from build123d import *

# Parameters (mm, degrees)
F0_W     = 15.85
F0_H     = 47.8
F1_DEPTH = 5
F2_R     = 2.5
F3_DEPTH = 2
F4_W     = 13.33
F4_H     = 44.9
F5_DEPTH = 2.8
F7_DEPTH = 2.8


with BuildPart() as f1:
    # F0 (on Top) → F1 (new body)
    with BuildSketch(Plane.XY):
        with Locations((-44.90279, 38.503254)):
            Rectangle(F0_W, F0_H)
    extrude(amount=F1_DEPTH)

    # F2 (on face) → F3 (join)
    with BuildSketch(Plane.XY.offset(5)):
        with Locations((-48.82779, 58.403254)):
            Circle(F2_R)
        with Locations((-40.97779, 58.403254)):
            Circle(F2_R)
        with Locations((-48.82779, 18.603254)):
            Circle(F2_R)
        with Locations((-40.97779, 18.603254)):
            Circle(F2_R)
        with Locations((-48.82779, 50.403254)):
            Circle(F2_R)
        with Locations((-40.97779, 50.403254)):
            Circle(F2_R)
        with Locations((-48.82779, 26.403254)):
            Circle(F2_R)
        with Locations((-40.97779, 26.403254)):
            Circle(F2_R)
        with Locations((-48.82779, 42.403254)):
            Circle(F2_R)
        with Locations((-40.97779, 42.403254)):
            Circle(F2_R)
        with Locations((-48.82779, 34.403254)):
            Circle(F2_R)
        with Locations((-40.97779, 34.403254)):
            Circle(F2_R)
    extrude(amount=F3_DEPTH)

    # F4 (on face) → F5 (cut)
    with BuildSketch(Plane(origin=(0, 0, 0), x_dir=(1, 0, 0), z_dir=(0, 0, -1))):
        with Locations((-44.856941, -38.523254)):
            Rectangle(F4_W, F4_H)
    extrude(amount=-F5_DEPTH, mode=Mode.SUBTRACT)

    # F6 (on face) → F7 (join)
    with BuildSketch(Plane(origin=(0, 0, 2.8), x_dir=(1, 0, 0), z_dir=(0, 0, -1))):
        with BuildLine():
            ThreePointArc((-41.606941, -21.923254), (-42.558844, -19.625157), (-44.856941, -18.673254))
            Line((-44.856941, -18.673254), (-44.856941, -19.873254))
            ThreePointArc((-44.856941, -19.873254), (-43.407372, -20.473685), (-42.806941, -21.923254))
            ThreePointArc((-42.806941, -21.923254), (-43.407372, -23.372823), (-44.856941, -23.973254))
            Line((-44.856941, -23.973254), (-44.856941, -25.173254))
            ThreePointArc((-44.856941, -25.173254), (-42.558844, -24.221351), (-41.606941, -21.923254))
        make_face()
        with BuildLine():
            ThreePointArc((-41.783448, -56.322801), (-42.673771, -54.08798), (-44.856941, -53.077598))
            Line((-44.856941, -53.077598), (-44.856941, -54.279652))
            ThreePointArc((-44.856941, -54.279652), (-43.516394, -54.933528), (-42.973804, -56.32285))
            ThreePointArc((-42.973804, -56.32285), (-43.516394, -57.712172), (-44.856941, -58.366047))
            Line((-44.856941, -58.366047), (-44.856941, -59.568005))
            ThreePointArc((-44.856941, -59.568005), (-42.673771, -58.557623), (-41.783448, -56.322801))
        make_face()
        with BuildLine():
            Line((-44.856941, -54.279652), (-44.856941, -53.077598))
            ThreePointArc((-44.856941, -53.077598), (-48.283448, -56.322801), (-44.856941, -59.568005))
            Line((-44.856941, -59.568005), (-44.856941, -58.366047))
            ThreePointArc((-44.856941, -58.366047), (-47.073804, -56.32285), (-44.856941, -54.279652))
        make_face()
        with BuildLine():
            ThreePointArc((-41.739321, -47.722915), (-42.644888, -45.472108), (-44.856941, -44.475612))
            Line((-44.856941, -44.475612), (-44.856941, -45.676774))
            ThreePointArc((-44.856941, -45.676774), (-43.488929, -46.318325), (-42.932089, -47.722951))
            ThreePointArc((-42.932089, -47.722951), (-43.488929, -49.127577), (-44.856941, -49.769127))
            Line((-44.856941, -49.769127), (-44.856941, -50.970217))
            ThreePointArc((-44.856941, -50.970217), (-42.644888, -49.973722), (-41.739321, -47.722915))
        make_face()
        with BuildLine():
            Line((-44.856941, -45.676774), (-44.856941, -44.475612))
            ThreePointArc((-44.856941, -44.475612), (-48.239321, -47.722915), (-44.856941, -50.970217))
            Line((-44.856941, -50.970217), (-44.856941, -49.769127))
            ThreePointArc((-44.856941, -49.769127), (-47.032089, -47.722951), (-44.856941, -45.676774))
        make_face()
        with BuildLine():
            ThreePointArc((-41.695195, -39.123028), (-42.616104, -36.856348), (-44.856941, -35.874226))
            Line((-44.856941, -35.874226), (-44.856941, -37.07475))
            ThreePointArc((-44.856941, -37.07475), (-43.461601, -37.703287), (-42.890373, -39.123052))
            ThreePointArc((-42.890373, -39.123052), (-43.461601, -40.542817), (-44.856941, -41.171353))
            Line((-44.856941, -41.171353), (-44.856941, -42.371829))
            ThreePointArc((-44.856941, -42.371829), (-42.616104, -41.389708), (-41.695195, -39.123028))
        make_face()
        with BuildLine():
            Line((-44.856941, -37.07475), (-44.856941, -35.874226))
            ThreePointArc((-44.856941, -35.874226), (-48.195195, -39.123028), (-44.856941, -42.371829))
            Line((-44.856941, -42.371829), (-44.856941, -41.171353))
            ThreePointArc((-44.856941, -41.171353), (-46.990373, -39.123052), (-44.856941, -37.07475))
        make_face()
        with BuildLine():
            ThreePointArc((-41.651068, -30.523141), (-42.587422, -28.240698), (-44.856941, -27.273441))
            Line((-44.856941, -27.273441), (-44.856941, -28.473578))
            ThreePointArc((-44.856941, -28.473578), (-43.434414, -29.088409), (-42.848657, -30.523153))
            ThreePointArc((-42.848657, -30.523153), (-43.434414, -31.957897), (-44.856941, -32.572729))
            Line((-44.856941, -32.572729), (-44.856941, -33.772842))
            ThreePointArc((-44.856941, -33.772842), (-42.587422, -32.805584), (-41.651068, -30.523141))
        make_face()
        with BuildLine():
            Line((-44.856941, -28.473578), (-44.856941, -27.273441))
            ThreePointArc((-44.856941, -27.273441), (-48.151068, -30.523141), (-44.856941, -33.772842))
            Line((-44.856941, -33.772842), (-44.856941, -32.572729))
            ThreePointArc((-44.856941, -32.572729), (-46.948657, -30.523153), (-44.856941, -28.473578))
        make_face()
        with BuildLine():
            Line((-44.856941, -19.873254), (-44.856941, -18.673254))
            ThreePointArc((-44.856941, -18.673254), (-48.106941, -21.923254), (-44.856941, -25.173254))
            Line((-44.856941, -25.173254), (-44.856941, -23.973254))
            ThreePointArc((-44.856941, -23.973254), (-46.906941, -21.923254), (-44.856941, -19.873254))
        make_face()
    extrude(amount=F7_DEPTH)


solid = f1.part
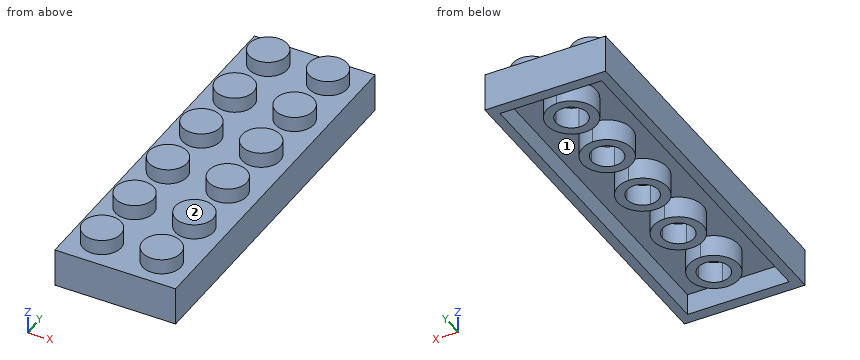
Geometry check sheet. Reference: the model listing, model coordinates, mm. Face numbers are marked on the shaded views. A direction names the side the tool comes from. Give positions to 0.01 mm unless a question says otherwise; leave off trailing zeros. Write each loop counter-clockwise with the first axis right and the second up, starting at its lowest first coordinate (ties: lowest second). Pieces come first, ordered by that corner, then holes.
1) Set-up check for the marked faces 1 and 2: record each of +Z, -Z, +X, -X, +Y, -Y from which the full face is reachable in a straight line by a thin tool's end or side.
Values follow:
face 1: -Z
face 2: +Z, +X, -X, +Y, -Y
2) Cross-section at D-D (y = 44). Record the boundary of the cut face in (x, z).
Values follow:
outline: (-52.83, 0) - (-51.52, 0) - (-51.52, 2.8) - (-38.19, 2.8) - (-38.19, 0) - (-36.98, 0) - (-36.98, 5) - (-39.05, 5) - (-39.05, 7) - (-42.9, 7) - (-42.9, 5) - (-46.9, 5) - (-46.9, 7) - (-50.75, 7) - (-50.75, 5) - (-52.83, 5) - close
3) Go/stop test with a flat-tipped pin: pin 1 Ø2 at (x, y) = (-45, 56) entering from -Z. Record where the tip stops, or that it passes through.
Values follow:
pin 1: stops at z = 2.8
4) Thickness scan on line 1 (X direction, y = 51.5, z = 2.25); line 2 (Y direction, x = -51, z = 6); line 3 (Y direction, x = -39.25, z = 2.75). Record the ranges inside material, lowest first.
Values follow:
line 1: x = -52.83 to -51.52, -38.19 to -36.98
line 2: y = 17.37 to 19.84, 25.17 to 27.64, 33.17 to 35.64, 41.17 to 43.64, 49.17 to 51.64, 57.17 to 59.64
line 3: y = 14.6 to 16.07, 60.97 to 62.4
5) Cross-section at A-A (z = 6). Count the separate pieces of the cut face and the enclosed holes in it, plus the area to 3 significant figures.
Values follow:
separate pieces: 12
enclosed holes: 0
area: 236 mm2
